Check sheet for the drawn part. Datum: minimum x, y, z corner. Units: mm. A direction names the side the tool comes from. Round coordinates to 2 decimals unless told otherwise and drop trailing zeros. Order: outer loops, then holes, each group sorted by start corner. A loop starts at its lowest first (then second) coordinate and runs counter-clockwise, first axis right, second up. Notation, with made-up numbers: (15, 58.5) -> (57, 58.5) arc R25 cw to (57, 90.5) -> close; hole circle Ø9 at (49.5, 32). An arc over 180 degrees is marked (long way). Answer as a JSON object with one key per item and string values. Group by question number.
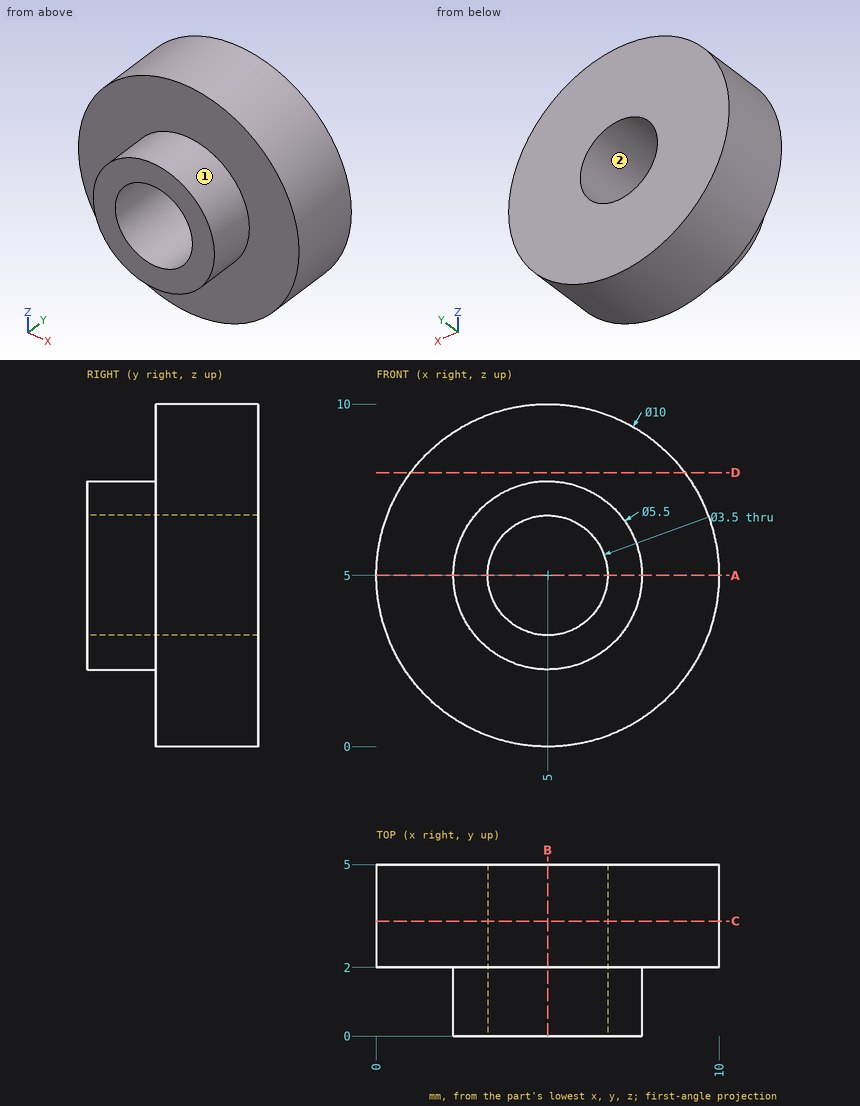
Item 1: Depth check by flat-ended pin: pin 1 Ø1.5 at (x, z) = (4.5, 1.5) entering from -Y; pin 2 Ø3 at (x, z) = (5, 5) entering from -Y; pin 3 Ø2 at (y, z) = (0.5, 6) entering from +X; pin 4 Ø1.5 at (x, y) = (2.5, 2) entering from +Z. Enter the tip coordinate at first touch or a pass-through.
Item 2: Set-up check for the marked faces 1 and 2: record each of +Z, -Z, +X, -X, +Y, -Y from which the full face is reachable in a straight line by a thin tool's end or side.
Item 3: Sectioned sample at D-D, the plane z = 8. Enter the section's corners in (x, y).
Item 4: Thickness scan on L1, parallel to X at y = 3.6, z = 5; L2, parallel to X at y = 1.35, z = 5. Record the ranges inside material, lowest first.
Item 5: Sectioned sample at A-A, the plane z = 5. Enter the section's corners in (x, y).
Item 6: Sectioned sample at B-B, the plane x = 5. Enter the section's corners in (y, z), then the cut area to 3 significant figures.
Item 7: Sectioned sample at C-C, the plane y = 3.35. Enter the section's corners in (x, z).
Result:
{
 "1": {"pin 1": "stops at y = 2", "pin 2": "passes through", "pin 3": "stops at x = 7.75", "pin 4": "stops at z = 9.68"},
 "2": {"face 1": "-Y", "face 2": "+Y, -Y"},
 "3": {"outline": "(1, 2) -> (9, 2) -> (9, 5) -> (1, 5) -> close"},
 "4": {"L1": "x = 0 to 3.25, 6.75 to 10", "L2": "x = 2.25 to 3.25, 6.75 to 7.75"},
 "5": {"outline": "(0, 2) -> (2.25, 2) -> (2.25, 0) -> (3.25, 0) -> (3.25, 5) -> (0, 5) -> close; (6.75, 0) -> (7.75, 0) -> (7.75, 2) -> (10, 2) -> (10, 5) -> (6.75, 5) -> close"},
 "6": {"outline": "(0, 2.25) -> (2, 2.25) -> (2, 0) -> (5, 0) -> (5, 3.25) -> (0, 3.25) -> close; (0, 6.75) -> (5, 6.75) -> (5, 10) -> (2, 10) -> (2, 7.75) -> (0, 7.75) -> close", "area": "23.5 mm2"},
 "7": {"outline": "circle Ø10 at (5, 5); hole circle Ø3.5 at (5, 5)"}
}
